Read the model definition and answer for the solid it produces. Units are mm, in the model's axes. Face numbers are marked on the shaded views. Coordinates: 2 decimals unless noted, no trailing zeros. Loops run counter-clockwise (first coordinate to the right, second up) from the corner with the lowest first, then second, coordinate; pieces in that order, holes last.
from build123d import *

# Parameters (mm, degrees)
SKETCH_1_W      = 72
SKETCH_1_H      = 20
SKETCH_1_R      = 2.1
EXTRUDE_1_DEPTH = 5


with BuildPart() as part:
    # 草图1 → 凸台-拉伸1 (new body)
    with BuildSketch(Plane.XZ.offset(5)):
        with Locations((0, 10)):
            Rectangle(SKETCH_1_W, SKETCH_1_H)
        with Locations(Location((10, 10, 0), (0, 0, 90))):
            Circle(SKETCH_1_R, mode=Mode.SUBTRACT)
        with Locations(Location((26, 10, 0), (0, 0, 90))):
            Circle(SKETCH_1_R, mode=Mode.SUBTRACT)
        with Locations(Location((-10, 10, 0), (0, 0, 90))):
            Circle(SKETCH_1_R, mode=Mode.SUBTRACT)
        with Locations(Location((-26, 10, 0), (0, 0, 90))):
            Circle(SKETCH_1_R, mode=Mode.SUBTRACT)
        with Locations(Location((0, 10, 0), (0, 0, 90))):
            Circle(SKETCH_1_R, mode=Mode.SUBTRACT)
    extrude(amount=-EXTRUDE_1_DEPTH)


solid = part.part
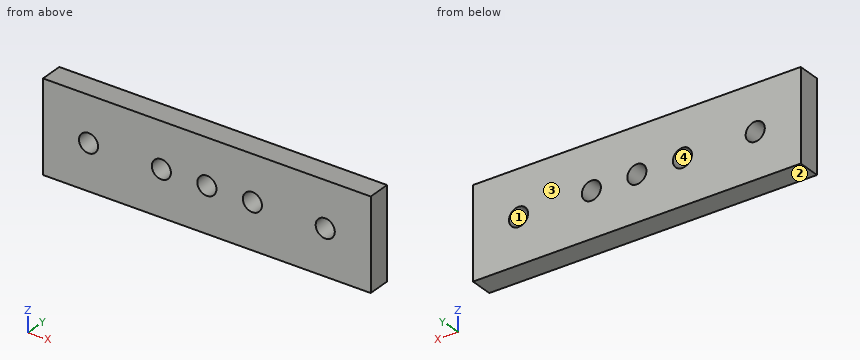
Q1. A cutting plane is placed at D-D (x = 9). Give the vertices of the cut face in (y, z).
Findings below:
outline: (-5, 0) - (0, 0) - (0, 8.15) - (-5, 8.15) - close; (-5, 11.85) - (0, 11.85) - (0, 20) - (-5, 20) - close
Q2. Determine the mould class of the marked faces 1, 2, 3 and 4 for opening direction Z: +Z half, -Z half, draft (parallel to the pull), parting line (faces both ways), or undercut.
Findings below:
face 1: undercut
face 2: -Z half
face 3: draft
face 4: undercut
Q3. A cutting plane is placed at A-A (z = 10). Give the vertices of the cut face in (x, y), then the cut area to 3 significant figures.
Findings below:
outline: (-36, -5) - (-28.1, -5) - (-28.1, 0) - (-36, 0) - close; (-23.9, -5) - (-12.1, -5) - (-12.1, 0) - (-23.9, 0) - close; (-7.9, -5) - (-2.1, -5) - (-2.1, 0) - (-7.9, 0) - close; (2.1, -5) - (7.9, -5) - (7.9, 0) - (2.1, 0) - close; (12.1, -5) - (23.9, -5) - (23.9, 0) - (12.1, 0) - close; (28.1, -5) - (36, -5) - (36, 0) - (28.1, 0) - close
area: 255 mm2
Q4. A cutting plane is placed at B-B (y = -0.9). Give the vertices of the cut face in (x, z), then the cut area to 3 significant figures.
Findings below:
outline: (-36, 0) - (36, 0) - (36, 20) - (-36, 20) - close; hole circle Ø4.2 at (-26, 10); hole circle Ø4.2 at (-10, 10); hole circle Ø4.2 at (0, 10); hole circle Ø4.2 at (10, 10); hole circle Ø4.2 at (26, 10)
area: 1,370 mm2
Q5. A cutting plane is placed at C-C (x = -10). Give the vertices of the cut face in (y, z).
Findings below:
outline: (-5, 0) - (0, 0) - (0, 7.9) - (-5, 7.9) - close; (-5, 12.1) - (0, 12.1) - (0, 20) - (-5, 20) - close
Q6. Straight lines are drawn through the part: probe 1 along X at (y, z) = (-3.6, 10); probe 2 along Z at (x, y) = (-26, -2.05); probe 3 along X at (y, z) = (-2.75, 8.5). For each, find the intervals that lie inside material, in ascending order.
Findings below:
probe 1: x = -36 to -28.1, -23.9 to -12.1, -7.9 to -2.1, 2.1 to 7.9, 12.1 to 23.9, 28.1 to 36
probe 2: z = 0 to 7.9, 12.1 to 20
probe 3: x = -36 to -27.47, -24.53 to -11.47, -8.53 to -1.47, 1.47 to 8.53, 11.47 to 24.53, 27.47 to 36
